from build123d import *

# Parameters (mm, degrees)
SKETCH5_W           = 73.577123652
SKETCH5_H           = 99.547402554
BOSS_EXTRUDE2_DEPTH = 50.8
SKETCH6_W           = 30.82640112
SKETCH6_H           = 95.25
CUT_EXTRUDE3_DEPTH  = 50.8
SKETCH7_W           = 37.670722532
SKETCH7_H           = 95.25
CUT_EXTRUDE4_DEPTH  = 50.8
SKETCH8_W           = 2.54
SKETCH8_H           = 84.265204652
BOSS_EXTRUDE3_DEPTH = 10.16
SKETCH9_W           = 2.649849203
SKETCH9_H           = 84.265204652
BOSS_EXTRUDE4_DEPTH = 10.16
SKETCH10_R          = 1.3048994
CUT_EXTRUDE5_DEPTH  = 10.16
SKETCH11_R          = 1.324924601
CUT_EXTRUDE6_DEPTH  = 10.16
SKETCH12_R          = 1.221520127
CUT_EXTRUDE7_DEPTH  = 10.16
SKETCH13_R          = 1.364093366
CUT_EXTRUDE8_DEPTH  = 10.16


with BuildPart() as part:
    # Sketch5 → Boss-Extrude2 (new body)
    with BuildSketch(Plane.XY):
        with Locations((36.788561826, 49.773701277)):
            Rectangle(SKETCH5_W, SKETCH5_H)
    extrude(amount=BOSS_EXTRUDE2_DEPTH)

    # Sketch6 → Cut-Extrude3 (cut)
    with BuildSketch(Plane.XY.offset(50.8)):
        with Locations((15.41320056, 51.922402554)):
            Rectangle(SKETCH6_W, SKETCH6_H)
    extrude(amount=-CUT_EXTRUDE3_DEPTH, mode=Mode.SUBTRACT)

    # Sketch7 → Cut-Extrude4 (cut)
    with BuildSketch(Plane.XY.offset(50.8)):
        with Locations((54.741762386, 51.922402554)):
            Rectangle(SKETCH7_W, SKETCH7_H)
    extrude(amount=-CUT_EXTRUDE4_DEPTH, mode=Mode.SUBTRACT)

    # Sketch8 → Boss-Extrude3 (add)
    with BuildSketch(Plane(origin=(35.90640112, 0, 0), x_dir=(0, 0, -1), z_dir=(1, 0, 0))):
        with Locations((-41.751497199, 51.694841949)):
            Rectangle(SKETCH8_W, SKETCH8_H)
    extrude(amount=BOSS_EXTRUDE3_DEPTH)

    # Sketch9 → Boss-Extrude4 (add)
    with BuildSketch(Plane(origin=(35.90640112, 0, 0), x_dir=(0, 0, -1), z_dir=(1, 0, 0))):
        with Locations((-14.668110729, 51.032379648)):
            Rectangle(SKETCH9_W, SKETCH9_H)
    extrude(amount=BOSS_EXTRUDE4_DEPTH)

    # Sketch10 → Cut-Extrude5 (cut)
    with BuildSketch(Plane(origin=(35.90640112, 0, 0), x_dir=(0, 0, -1), z_dir=(1, 0, 0))):
        with Locations((-45.406361482, 72.363665732)):
            Circle(SKETCH10_R)
    extrude(amount=-CUT_EXTRUDE5_DEPTH, mode=Mode.SUBTRACT)

    # Sketch11 → Cut-Extrude6 (cut)
    with BuildSketch(Plane(origin=(35.90640112, 0, 0), x_dir=(0, 0, -1), z_dir=(1, 0, 0))):
        with Locations((-10.958321844, 73.158620492)):
            Circle(SKETCH11_R)
    extrude(amount=-CUT_EXTRUDE6_DEPTH, mode=Mode.SUBTRACT)

    # Sketch12 → Cut-Extrude7 (cut)
    with BuildSketch(Plane(origin=(35.90640112, 0, 0), x_dir=(0, 0, -1), z_dir=(1, 0, 0))):
        with Locations((-46.201316243, 33.013405069)):
            Circle(SKETCH12_R)
    extrude(amount=-CUT_EXTRUDE7_DEPTH, mode=Mode.SUBTRACT)

    # Sketch13 → Cut-Extrude8 (cut)
    with BuildSketch(Plane(origin=(35.90640112, 0, 0), x_dir=(0, 0, -1), z_dir=(1, 0, 0))):
        with Locations((-11.355799225, 30.893525706)):
            Circle(SKETCH13_R)
    extrude(amount=-CUT_EXTRUDE8_DEPTH, mode=Mode.SUBTRACT)


solid = part.part
The model under review builds one solid part; all positions refer to its coordinate system, in mm. A direction names the side the tool comes from. Give positions to 0.01 mm unless a question says otherwise; leave off trailing zeros. Order: outer loops, then holes, each group sorted by start corner. A loop starts at its lowest first (then second) coordinate and runs counter-clockwise, first axis right, second up. Notation, with made-up numbers: M -20.5,-29 L 36.5,-29 A31 cw 36.5,2 Z; hole C -1,54 d2. An arc over 180 degrees is marked long. Use one line per item in the form item = value. Start each with the question number.
Item 1: For faces 1 (the flat face through (41, 50, 15.993)), 2 (the flat face through (30.826, 51, 26)), 3 (the flat face through (46.066, 52, 42)), list the 3-axis set-ups (+Z, -Z, +X, -X, +Y, -Y) from which the entire face can be reached by the end or side of a thin tool; tool diameter is ignored.
Item 2: We need section B-B on y = 41. Give the boundary of the cut face in (x, z), plus the area to 3 significant figures.
Item 3: We need section C-C on z = 39. Give the boundary of the cut face in (x, y), plus the area to 3 significant figures.
Item 4: Insertion check: pin 1 Ø3 at (y, z) = (47, 15) entering from +X; pin 2 Ø3 at (y, z) = (72.36, 45.41) entering from -X; pin 3 Ø1.3 at (x, z) = (41.5, 42) entering from +Y; pin 4 Ø2 at (y, z) = (33.01, 46.2) entering from -X. Each pin has a flat end and moves straight along its axis. Give the tip position at first contact, or say it passes through.
Item 5: The part is to be moulded in two halves that separate along Z. For faces 4 (the flat face through (34, 35, 0)), 5 (the cylindrical face through (33.4, 31.82, 46.47)), 6 (the flat face through (41, 51, 43.021)), 7 (the flat face through (46.066, 52, 15)), say which applies: pulls with the +Z half, pulls with the -Z half, needs draft (parallel to the pull), parting line crosses it, or undercut.
Item 6: We need section D-D on x = 4.5. Give the boundary of the cut face in (y, z), plus the area to 3 significant figures.
Item 7: To check wall thickness, follow line 1 along Z through (x, y) = (37, 15.5); line 2 along X through (y, z) = (84.5, 13); line 3 along Y through (x, z) = (63.5, 33.5). State the ranges of each line that lie inside material, in increasing order. Write a range as from..to.
Item 8: We need section A-A on x = 40. Give the boundary of the cut face in (y, z), plus the area to 3 significant figures.
Completed:
q1.face_1 = +X, +Y
q1.face_2 = +Z, -Z, -X, +Y
q1.face_3 = +Z, -Z, +X, +Y
q2.outline = M 30.83,0 L 35.91,0 L 35.91,13.34 L 46.07,13.34 L 46.07,15.99 L 35.91,15.99 L 35.91,40.48 L 46.07,40.48 L 46.07,43.02 L 35.91,43.02 L 35.91,50.8 L 30.83,50.8 Z
q2.area = 311 mm²
q3.outline = M 0,0 L 73.58,0 L 73.58,4.3 L 35.91,4.3 L 35.91,99.55 L 30.83,99.55 L 30.83,4.3 L 0,4.3 Z
q3.area = 800 mm²
q4.pin_1 = 46.07
q4.pin_2 = 30.83
q4.pin_3 = 93.83
q4.pin_4 = through
q5.face_4 = pulls with the -Z half
q5.face_5 = undercut
q5.face_6 = pulls with the +Z half
q5.face_7 = needs draft
q6.outline = M 0,0 L 4.3,0 L 4.3,50.8 L 0,50.8 Z
q6.area = 218 mm²
q7.line_1 = 13.34..15.99, 40.48..43.02
q7.line_2 = 30.83..35.91
q7.line_3 = 0..4.3
q8.outline = M 0,0 L 4.3,0 L 4.3,50.8 L 0,50.8 Z; M 8.9,13.34 L 93.16,13.34 L 93.16,15.99 L 8.9,15.99 Z; M 9.56,40.48 L 93.83,40.48 L 93.83,43.02 L 9.56,43.02 Z
q8.area = 656 mm²
